Autodesk Inventor part; units mm, degrees
ref_plane "YZ Plane" through (0, 0, 0) normal (1, 0, 0) x (0, 1, 0)
ref_plane "XZ Plane" through (0, 0, 0) normal (0, 1, 0) x (-1, 0, 0)
ref_plane "XY Plane" through (0, 0, 0) normal (0, 0, 1) x (1, 0, 0)
sketch "Sketch1" plane through (0, 0, 0) normal (0, 1, 0) x (-1, 0, 0)
  line L0 (50, 30.5) -> (-50, 30.5)
  line L1 (-50, 30.5) -> (-50, -30.5)
  line L2 (-50, -30.5) -> (50, -30.5)
  line L3 (50, -30.5) -> (50, 30.5)
  line L4 (50, 30.5) -> (-50, -30.5) construction
  line L5 (-50, 30.5) -> (50, -30.5) construction
  point P0 (0, 0)
  dimension "d4" = 61
  dimension "d5" = 100
extrude "Extrusion1" add sketch "Sketch1" along normal blind 5
sketch "Sketch2" plane through (0, 5, 0) normal (0, 1, 0) x (1, 0, 0)
  point P0 (0, 0)
hole "Hole1" at (0, 5, 0) direction (0, -1, 0) diameter 8 end up to surface
properties part number "jalador"
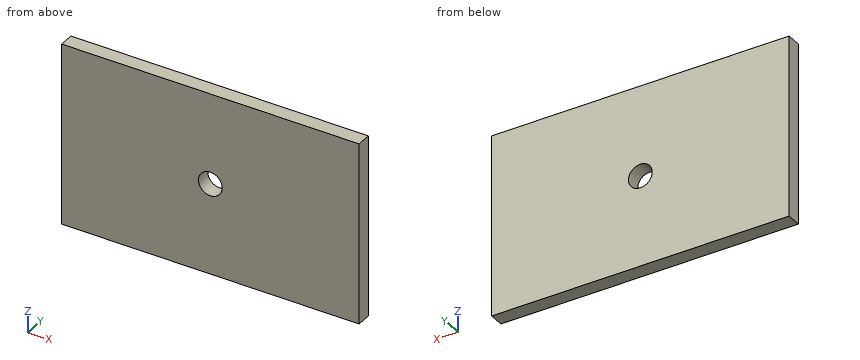
Read the model definition and answer for the solid it produces. Units are mm, in the model's axes. Give positions to 0.01 mm unless a question says otherwise; leave off trailing zeros. Order: outer loops, then holes, each group sorted by start corner. A loop starts at its lowest first (then second) coordinate and runs counter-clockwise, first axis right, second up. Notation, with made-up numbers: (53.25, -36.5) -> (93.25, -36.5) arc R33 ccw to (93.25, 0.5) -> close; hole circle Ø9 at (48, 79). An arc over 180 degrees is marked (long way). One line per item, written item: value. Start each with the question number.
(1) A flat-ended cylindrical pin translates along its axis: P1, Ø6.5, axis at x = 0, z = 0, coming from the -Y side. Find the tip coordinate at first contact, or state that the pin passes through.
(2) The part is cut by section B-B (x = 0). Determine the outline of the cut face in (y, z).
(3) Straight lines are drawn through the part: L1, parallel to X at y = 3.1, z = 0; L2, parallel to Z at x = 0, y = 3.55; L3, parallel to X at y = 0.8, z = 3. For each, find the intervals that lie inside material, in ascending order.
(4) The part is cut by section A-A (z = 0). Determine the outline of the cut face in (x, y), and give its area (3 significant figures).
Taken from the geometry:
1. P1: through
2. outline: (0, -30.5) -> (5, -30.5) -> (5, -4) -> (0, -4) -> close; (0, 4) -> (5, 4) -> (5, 30.5) -> (0, 30.5) -> close
3. L1: -50 to -4, 4 to 50
3. L2: -30.5 to -4, 4 to 30.5
3. L3: -50 to -2.65, 2.65 to 50
4. outline: (-50, 0) -> (-4, 0) -> (-4, 5) -> (-50, 5) -> close; (4, 0) -> (50, 0) -> (50, 5) -> (4, 5) -> close
4. area: 460 mm^2
